Model file for the job. Use its own axes, mm. A direction names the side the tool comes from. Round coordinates to 2 decimals unless told otherwise and drop trailing zeros. Loops run counter-clockwise (first coordinate to the right, second up) from the corner with the lowest first, then second, coordinate; pieces in that order, holes last.
from build123d import *

# Parameters (mm, degrees)
MODEL_R                 = 8
MODEL_R_2               = 6
SALIENTE_EXTRUIR1_DEPTH = 3


with BuildPart() as part:
    # Model → Saliente-Extruir1 (new body)
    with BuildSketch(Plane.XY):
        with BuildLine():
            Line((30.519021416, 15.672169472), (30.519021416, -38.327830528))
            ThreePointArc((30.519021416, -38.327830528), (30.226128197, -39.034937309), (29.519021416, -39.327830528))
            Line((29.519021416, -39.327830528), (21.519021416, -39.327830528))
            ThreePointArc((21.519021416, -39.327830528), (20.811914634, -39.620723747), (20.519021416, -40.327830528))
            Line((20.519021416, -40.327830528), (20.519021416, -62.327830528))
            ThreePointArc((20.519021416, -62.327830528), (20.226128197, -63.034937309), (19.519021416, -63.327830528))
            Line((19.519021416, -63.327830528), (9.355410048, -63.327830528))
            Line((9.355410048, -63.327830528), (9.355410048, -59.327830528))
            Line((9.355410048, -59.327830528), (6.355410048, -59.327830528))
            Line((6.355410048, -59.327830528), (6.355410048, -63.327830528))
            Line((6.355410048, -63.327830528), (3.355410048, -63.327830528))
            ThreePointArc((3.355410048, -63.327830528), (2.648303267, -63.034937309), (2.355410048, -62.327830528))
            Line((2.355410048, -62.327830528), (2.355410048, -40.327830528))
            ThreePointArc((2.355410048, -40.327830528), (2.062516829, -39.620723747), (1.355410048, -39.327830528))
            Line((1.355410048, -39.327830528), (-6.644589952, -39.327830528))
            ThreePointArc((-6.644589952, -39.327830528), (-7.351696733, -39.620723747), (-7.644589952, -40.327830528))
            Line((-7.644589952, -40.327830528), (-7.644589952, -62.327830528))
            ThreePointArc((-7.644589952, -62.327830528), (-7.937483171, -63.034937309), (-8.644589952, -63.327830528))
            Line((-8.644589952, -63.327830528), (-11.644589952, -63.327830528))
            Line((-11.644589952, -63.327830528), (-11.644589952, -59.327830528))
            Line((-11.644589952, -59.327830528), (-14.644589952, -59.327830528))
            Line((-14.644589952, -59.327830528), (-14.644589952, -63.327830528))
            Line((-14.644589952, -63.327830528), (-24.80820132, -63.327830528))
            ThreePointArc((-24.80820132, -63.327830528), (-25.515308101, -63.034937309), (-25.80820132, -62.327830528))
            Line((-25.80820132, -62.327830528), (-25.80820132, -40.549556443))
            ThreePointArc((-25.80820132, -40.549556443), (-26.101094538, -39.842449662), (-26.80820132, -39.549556443))
            Line((-26.80820132, -39.549556443), (-34.80820132, -39.549556443))
            ThreePointArc((-34.80820132, -39.549556443), (-35.515308101, -39.256663224), (-35.80820132, -38.549556443))
            Line((-35.80820132, -38.549556443), (-35.80820132, 8.978477483))
            Line((-35.80820132, 8.978477483), (-35.80820132, 15.672169472))
            ThreePointArc((-35.80820132, 15.672169472), (-35.515308101, 16.379276253), (-34.80820132, 16.672169472))
            Line((-34.80820132, 16.672169472), (-21.80820132, 16.672169472))
            ThreePointArc((-21.80820132, 16.672169472), (-21.101094538, 16.965062691), (-20.80820132, 17.672169472))
            Line((-20.80820132, 17.672169472), (-20.80820132, 20.672169472))
            ThreePointArc((-20.80820132, 20.672169472), (-21.101094538, 21.379276253), (-21.80820132, 21.672169472))
            Line((-21.80820132, 21.672169472), (-35.80820132, 21.672169472))
            Line((-35.80820132, 21.672169472), (-31.000008461, 51.449360761))
            ThreePointArc((-31.000008461, 51.449360761), (-30.856229997, 52.641077199), (-30.80820132, 53.840474364))
            Line((-30.80820132, 53.840474364), (-30.80820132, 69.672169472))
            ThreePointArc((-30.80820132, 69.672169472), (-26.414803037, 80.27877119), (-15.80820132, 84.672169472))
            Line((-15.80820132, 84.672169472), (10.519021416, 84.672169472))
            ThreePointArc((10.519021416, 84.672169472), (21.125623133, 80.27877119), (25.519021416, 69.672169472))
            Line((25.519021416, 69.672169472), (25.519021416, 62.471272593))
            Line((25.519021416, 62.471272593), (25.519021416, 53.840474364))
            ThreePointArc((25.519021416, 53.840474364), (25.567050093, 52.641077199), (25.710828557, 51.449360761))
            Line((25.710828557, 51.449360761), (30.519021416, 21.672169472))
            Line((30.519021416, 21.672169472), (16.519021416, 21.672169472))
            ThreePointArc((16.519021416, 21.672169472), (15.811914634, 21.379276253), (15.519021416, 20.672169472))
            Line((15.519021416, 20.672169472), (15.519021416, 17.672169472))
            ThreePointArc((15.519021416, 17.672169472), (15.811914634, 16.965062691), (16.519021416, 16.672169472))
            Line((16.519021416, 16.672169472), (29.519021416, 16.672169472))
            ThreePointArc((29.519021416, 16.672169472), (30.226128197, 16.379276253), (30.519021416, 15.672169472))
        make_face()
        with Locations((-15.644589952, 61.620749462)):
            Circle(MODEL_R, mode=Mode.SUBTRACT)
        with Locations((10.355410048, 61.620749462)):
            Circle(MODEL_R, mode=Mode.SUBTRACT)
        with Locations((-2.644589952, 42.420749462)):
            Circle(MODEL_R_2, mode=Mode.SUBTRACT)
        with BuildLine():
            Line((4.355410048, 22.420749462), (5.535659362, 22.420749462))
            ThreePointArc((5.535659362, 22.420749462), (6.488784367, 23.118172652), (6.112446409, 24.23764401))
            Line((6.112446409, 24.23764401), (4.355410048, 25.879525262))
            Line((4.355410048, 25.879525262), (4.355410048, 22.420749462))
        make_face(mode=Mode.SUBTRACT)
        Polygon((2.355410048, 22.420749462), (0.355410048, 22.420749462), (0.355410048, 29.617367662), (2.355410048, 27.748446462), align=None, mode=Mode.SUBTRACT)
        Polygon((-3.644589952, 31.486288862), (-2.644589952, 32.420749462), (-1.644589952, 31.486288862), (-1.644589952, 22.420749462), (-3.644589952, 22.420749462), align=None, mode=Mode.SUBTRACT)
        Polygon((-5.644589952, 22.420749462), (-7.644589952, 22.420749462), (-7.644589952, 27.748446462), (-5.644589952, 29.617367662), align=None, mode=Mode.SUBTRACT)
        with BuildLine():
            Line((-9.644589952, 22.420749462), (-10.824839266, 22.420749462))
            ThreePointArc((-10.824839266, 22.420749462), (-11.777964271, 23.118172652), (-11.401626313, 24.23764401))
            Line((-11.401626313, 24.23764401), (-9.644589952, 25.879525262))
            Line((-9.644589952, 25.879525262), (-9.644589952, 22.420749462))
        make_face(mode=Mode.SUBTRACT)
        Polygon((13.355410048, -33.327830528), (-18.644589952, -33.327830528), (-18.644589952, -1.327830528), (-2.144589952, -1.327830528), (13.355410048, -1.327830528), align=None, mode=Mode.SUBTRACT)
    extrude(amount=SALIENTE_EXTRUIR1_DEPTH)


solid = part.part
Q1. Pull direction X, two halves, no side cores. Call faces 1 (the face through (-2, 12, 3)), 2 (the face through (9.355, -61, 1)), 3 (the face through (-11.645, -61, 1)), 4 (the face through (-26.53, 80.16, 1.48)): pulls with the +X half, pulls with the -X half, needs draft (parallel to the pull), parting line crosses it, or undercut.
Q2. Flat gauge pins, fed straight in: P1, Ø0.9, axis at y = -54.5, z = 2, coming from the +X side; P2, Ø1.5, axis at x = -31, z = 1.5, coming from the -Y side; P3, Ø0.9, axis at y = 23.5, z = 1, coming from the -X side. Where does each tip first touch, or does it go through?
Q3. Tool access for faces 5 (the face through (-25.808, -52, 1)), 6 (the face through (2.355, 25, 1)), 7 (the face through (-3, -39.328, 1)), 8 (the face through (-29, 21.672, 1)): list every direction of +Z, -Z, +X, -X, +Y, -Y with a clear straight run to the whole face (end or side of a thin tool).
Q4. Probe line 1 (X direction, y = -42.5, z = 2.75); line 2 (Y direction, x = 12, z = 1.15); line 3 (X direction, y = -21.5, z = 1.95). List the from-to ranges inside material, lowest first.
Q5. Slice it at A-A on y = -5.5. Give the cut face in (x, z), plus the area to 3 significant figures.
Q6. Slice it at B-B on y = 64. Give the cut face in (x, z).
Q7. Slice it at D-D on x = 24. Give the cut face in (y, z), plus the area to 3 significant figures.
Q8. Slice it at C-C on x = 8. Give the cut face in (y, z), plus the area to 3 significant figures.
Reply:
1. face 1: needs draft
1. face 2: undercut
1. face 3: undercut
1. face 4: pulls with the -X half
2. P1: stops at x = 20.52
2. P2: stops at y = -39.55
2. P3: stops at x = -35.59
3. face 5: +Z, -Z, -X, -Y
3. face 6: +Z, -Z
3. face 7: +Z, -Z, -Y
3. face 8: +Z, -Z, -X
4. line 1: x = -25.81 to -7.64, 2.36 to 20.52
4. line 2: y = -63.33 to -33.33, -1.33 to 53.79, 69.45 to 84.6
4. line 3: x = -35.81 to -18.64, 13.36 to 30.52
5. outline: (-35.81, 0) - (-18.64, 0) - (-18.64, 3) - (-35.81, 3) - close; (13.36, 0) - (30.52, 0) - (30.52, 3) - (13.36, 3) - close
5. area: 103 mm2
6. outline: (-30.81, 0) - (-23.28, 0) - (-23.28, 3) - (-30.81, 3) - close; (-8.01, 0) - (2.72, 0) - (2.72, 3) - (-8.01, 3) - close; (17.99, 0) - (25.52, 0) - (25.52, 3) - (17.99, 3) - close
7. outline: (-39.33, 0) - (16.67, 0) - (16.67, 3) - (-39.33, 3) - close; (21.67, 0) - (76.25, 0) - (76.25, 3) - (21.67, 3) - close
7. area: 332 mm2
8. outline: (-59.33, 0) - (-33.33, 0) - (-33.33, 3) - (-59.33, 3) - close; (-1.33, 0) - (53.98, 0) - (53.98, 3) - (-1.33, 3) - close; (69.27, 0) - (84.67, 0) - (84.67, 3) - (69.27, 3) - close
8. area: 290 mm2
